from build123d import *

# Parameters (mm, degrees)
SKETCH1_R             = 11
SKETCH1_R_2           = 9.5
BOSS_EXTRUDE1_DEPTH   = 3.5
SKETCH1_R_3           = 5.5
SKETCH1_R_4           = 4
BOSS_EXTRUDE1_2_DEPTH = 3.5
SKETCH1_3_R           = 9.5
SKETCH1_3_R_2         = 5.5
BOSS_EXTRUDE2_DEPTH   = 3
CHAMFER1_SIZE         = 0.5


with BuildPart() as part:
    # Sketch1 → Boss-Extrude1 (new, symmetric)
    with BuildSketch(Plane.XY):
        Circle(SKETCH1_R)
        Circle(SKETCH1_R_2, mode=Mode.SUBTRACT)
    extrude(amount=BOSS_EXTRUDE1_DEPTH, both=True)



with BuildPart() as body_2:
    # Sketch1 → Boss-Extrude1 2 (new, symmetric)
    with BuildSketch(Plane.XY):
        Circle(SKETCH1_R_3)
        Circle(SKETCH1_R_4, mode=Mode.SUBTRACT)
    extrude(amount=BOSS_EXTRUDE1_2_DEPTH, both=True)


with BuildPart() as part_1:
    add(part.part)

    add(body_2.part)  # Boss-Extrude2 merges body 2
    # Sketch1<3> → Boss-Extrude2 (add, symmetric)
    with BuildSketch(Plane.XY):
        Circle(SKETCH1_3_R)
        Circle(SKETCH1_3_R_2, mode=Mode.SUBTRACT)
    extrude(amount=BOSS_EXTRUDE2_DEPTH, both=True)

    # Chamfer1
    chamfer1_edges = [part_1.edges().sort_by_distance(p)[0] for p in [
        (-5.5, 0, -3.5),
        (-5.5, 0, 3.5),
        (-11, 0, -3.5),
        (-11, 0, 3.5),
    ]]
    chamfer(chamfer1_edges, length=CHAMFER1_SIZE - 0.0001)  # a hair under: the kernel refuses the full size


solid = part_1.part
Build history of the part. All positions in model axes, mm. A direction names the side the tool comes from. Coordinates: 2 decimals unless noted, no trailing zeros. Order: outer loops, then holes, each group sorted by start corner. A loop starts at its lowest first (then second) coordinate and runs counter-clockwise, first axis right, second up. Notation, with made-up numbers: M 49,69 L 61,69 A13 ccw 61,93 Z; hole C -20.5,-12 d5. An arc over 180 degrees is marked long. One line per question, with ' | ' between items. Start each with the question number.
Q1. Flat gauge pins, fed straight in: pin 1 Ø3 at (y, z) = (8, 2.5) entering from +X; pin 2 Ø1 at (x, z) = (-4, -2.5) entering from -Y; pin 3 Ø1 at (x, y) = (-0.5, -7) entering from -Z. Where does each tip first touch, or does it go through?
Q2. Probe L1, parallel to Y at x = 0, z = -3.35; L2, parallel to Y at x = 0, z = -0.5; L3, parallel to Z at x = 7.5, y = -5.5. List the from-to ranges inside material, lowest first. Write a range as from..to.
Q3. Saw through at C-C (z = -1.75). List the corners of the cut face in (x, y), then the cut area to 3 significant figures.
Q4. 3-axis set-ups, long thin cutter, end or side, ignore diameter. For faces 1 (the face through (4, -4, -3)), 2 (the face through (-5, -9, 3.5)): which of +Z, -Z, +X, -X, +Y, -Y reach the whole face in a straight line?
Q5. Two-plate mould, pull along X, no slides. Class faces 3 (the face through (4, -4, 3)), 4 (the face through (-5, -9, -3.5)), 5 (the face through (4.38, -8.43, 3.25)), 6 (the face through (-2.38, -10.74, 0.04)): +X half, -X half, draft (parallel to the pull), parting line (faces both ways), or undercut.
Check values:
1) pin 1: stops at x = 8.87 | pin 2: stops at y = -10.43 | pin 3: stops at z = -3
2) L1: y = -10.65..-9.5, -5.15..-4, 4..5.15, 9.5..10.65 | L2: y = -11..-4, 4..11 | L3: z = -3..3
3) outline: C 0,0 d22; hole C 0,0 d8 | area: 330 mm2
4) face 1: -Z | face 2: +Z, +X, -X, +Y, -Y
5) face 3: undercut | face 4: draft | face 5: undercut | face 6: parting line
